The model under review builds one solid part; all positions refer to its coordinate system, in mm. A direction names the side the tool comes from. Coordinates: 2 decimals unless noted, no trailing zeros. Order: outer loops, then holes, each group sorted by start corner. A loop starts at its lowest first (then second) coordinate and runs counter-clockwise, first axis right, second up. Notation, with made-up numbers: (44.5, 80.5) -> (52.5, 80.5) arc R29 ccw to (52.5, 114.5) -> close; hole circle Ø6 at (-24, -19.5). An arc over 180 degrees is marked (long way). Use one line per item in the form item = value.
from build123d import *

# Parameters (mm, degrees)
EXTRUDE_THIN1_DEPTH = 254
FILLET1_R           = 1.27


with BuildPart() as part:
    # Sketch1 → Extrude-Thin1 (new body)
    with BuildSketch(Plane.XY):
        with BuildLine():
            Line((0, 0), (0, -3.175))
            Line((0, -3.175), (-4.7625, -3.175))
            ThreePointArc((-4.7625, -3.175), (-7.743674429, 7.852127417), (-15.875, 15.875))
            Line((-15.875, 15.875), (-15.875, 22.225))
            Line((-15.875, 22.225), (0, 22.225))
            Line((0, 22.225), (0, 19.05))
            Line((0, 19.05), (-1.27, 19.05))
            Line((-1.27, 19.05), (-1.27, 20.955))
            Line((-1.27, 20.955), (-14.605, 20.955))
            Line((-14.605, 20.955), (-14.605, 16.601962608))
            ThreePointArc((-14.605, 16.601962608), (-6.779670812, 8.71710723), (-3.527354833, -1.905))
            Line((-3.527354833, -1.905), (-1.27, -1.905))
            Line((-1.27, -1.905), (-1.27, 0))
            Line((-1.27, 0), (0, 0))
        make_face()
    extrude(amount=-EXTRUDE_THIN1_DEPTH)

    # Fillet1
    fillet1_edges = [part.edges().sort_by_distance(p)[0] for p in [
        (0, -3.175, -127),
        (-4.7625, -3.175, -127),
        (-15.875, 15.875, -127),
        (-15.875, 22.225, -127),
        (0, 22.225, -127),
    ]]
    fillet(fillet1_edges, radius=FILLET1_R)


solid = part.part
Item 1: We need section A-A (x = -8). Write out the cut boundary in (y, z) (3 decimals).
Results found:
outline = (8.28, -254) -> (10.552, -254) -> (10.552, 0) -> (8.28, 0) -> close; (20.955, -254) -> (22.225, -254) -> (22.225, 0) -> (20.955, 0) -> close
Item 2: We need section D-D (y = 2.5). Write out the cut boundary in (x, z), plus the area to 3 significant figures.
Results found:
outline = (-5.51, -254) -> (-4.2, -254) -> (-4.2, 0) -> (-5.51, 0) -> close
area = 333 mm²
Item 3: Draft analysis for pull direction X (two halves, no side actions). For faces 1 (the face through (-8.5, 10.5, 0)), 2 (the face through (-15.875, 19, -125)), 3 (the face through (-8, 20.955, -125)), state which applies: released by +X, released by -X, zero draft, split by the parting line, or undercut.
Results found:
face_1 = zero draft
face_2 = released by -X
face_3 = undercut
Item 4: To check wall thickness, follow L1, parallel to Y at x = -3.25, z = -58 (3 decimals); L2, parallel to X at y = 19.75, z = -9.5 (3 decimals); L3, parallel to X at y = -2, z = -81. State the ranges of each line that lie inside material, in increasing order. Write a range as from..to.
Results found:
L1 = -3.175..-1.905, 20.955..22.225
L2 = -15.875..-14.605, -1.27..0
L3 = -4.79..0
Item 5: Tool access review of faces 4 (the face through (-14.605, 19, -125)), 5 (the face through (-8, 22.225, -125)): name each direction out of +Z, -Z, +X, -X, +Y, -Y from which nothing blocks a thin tool from reaching the whole face with its end or side.
Results found:
face_4 = +Z, -Z
face_5 = +Z, -Z, +X, -X, +Y
Item 6: We need section C-C (y = 13). Write out the cut boundary in (x, z).
Results found:
outline = (-11.91, -254) -> (-10.08, -254) -> (-10.08, 0) -> (-11.91, 0) -> close
Item 7: Clearance check with flat-ended pins moving along their axes: pin 1 (6 mm diameter, centred on y = 11.5, z = -178.5, fed in from +X); pin 2 (1 mm diameter, centred on x = -0.5, z = -138.5, fed in from +Y); pin 3 (4 mm diameter, centred on x = -9, z = -102.5, fed in from -Y). State where each tip first meets the part, or that it passes through.
Results found:
pin_1 = -6.65
pin_2 = 22.2
pin_3 = 6.46
